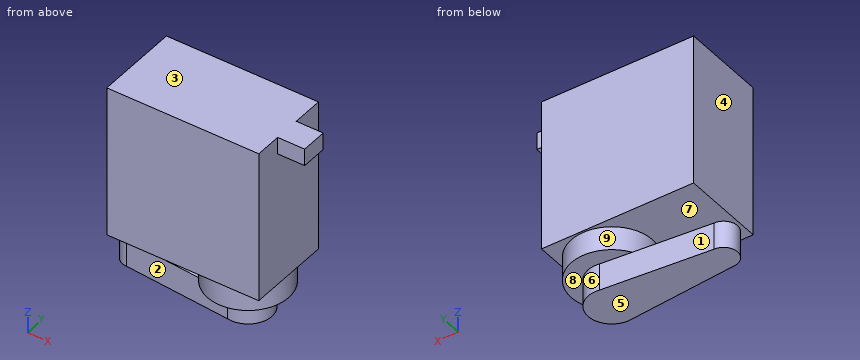
```python
from build123d import *

# Parameters (mm, degrees)
SKETCH1_W           = 22.5
SKETCH1_H           = 12.5
BOSS_EXTRUDE1_DEPTH = 22.5
SKETCH2_R           = 6
BOSS_EXTRUDE2_DEPTH = 3.5
BOSS_EXTRUDE4_DEPTH = 4
SKETCH6_W           = 2.526093831
SKETCH6_H           = 3.888015028
BOSS_EXTRUDE5_DEPTH = 4


with BuildPart() as part:
    # Sketch1 → Boss-Extrude1 (new body)
    with BuildSketch(Plane.XY):
        Rectangle(SKETCH1_W, SKETCH1_H)
    extrude(amount=BOSS_EXTRUDE1_DEPTH)

    # Sketch2 → Boss-Extrude2 (add)
    with BuildSketch(Plane(origin=(0, 0, 0), x_dir=(-1, 0, 0), z_dir=(0, 0, -1))):
        with Locations((-5.25, 0)):
            Circle(SKETCH2_R)
    extrude(amount=BOSS_EXTRUDE2_DEPTH)

    # Sketch5 → Boss-Extrude4 (add)
    with BuildSketch(Plane(origin=(0, 0, -3.5), x_dir=(-1, 0, 0), z_dir=(0, 0, -1))):
        with BuildLine():
            Line((-4.635129487, 3.455724852), (11.29, 2.05))
            ThreePointArc((11.29, 2.05), (13.34, 0), (11.29, -2.05))
            Line((11.29, -2.05), (-4.635129487, -3.455724852))
            ThreePointArc((-4.635129487, -3.455724852), (-8.76, 0), (-4.635129487, 3.455724852))
        make_face()
    extrude(amount=BOSS_EXTRUDE4_DEPTH)

    # Sketch6 → Boss-Extrude5 (add)
    with BuildSketch(Plane(origin=(11.25, 0, 0), x_dir=(0, 0, -1), z_dir=(1, 0, 0))):
        with Locations((-21.236953085, -0.353333214)):
            Rectangle(SKETCH6_W, SKETCH6_H)
    extrude(amount=BOSS_EXTRUDE5_DEPTH)


solid = part.part
```
The model under review builds one solid part; all positions refer to its coordinate system, in mm. Face numbers are marked on the shaded views. A direction names the side the tool comes from. Round coordinates to 2 decimals unless told otherwise and drop trailing zeros. Loops run counter-clockwise (first coordinate to the right, second up) from the corner with the lowest first, then second, coordinate; pieces in that order, holes last. Notation, with made-up numbers: (89.5, 42) - (94.5, 42) arc R30 ccw to (94.5, 72) - close; hole circle Ø6 at (58.25, -33.5). An arc over 180 degrees is marked (long way). Write each question's results on one line, items separated by ' | '. Start each with the question number.
Q1. Take a section at D-D on x = 10. Give the boundary of the cut face in (y, z).
Q2. Take a section at A-A on x = -2.75. Give the boundary of the cut face in (y, z), plus the area to 3 significant figures.
Q3. Wall thickness on line 1 along Z through (x, y) = (-6.5, -0.25); line 2 along X through (y, z) = (1.75, 13); line 3 along Z through (x, y) = (-10.25, 2.25): over which ranges is each line inside the solid? List them lowest first. Write a range as [from, to].
Q4. Draft analysis for pull direction Z (two halves, no side actions). For the marked faces 6, 7, 8 and 9, state which applies: pulls with the +Z half, pulls with the -Z half, needs draft (parallel to the pull), parting line crosses it, or undercut.
Q5. Take a section at B-B on z = 2. Give the boundary of the cut face in (x, y).
Q6. Tool access review of the marked faces 1, 2, 3, 4 and 5: name each direction out of +Z, -Z, +X, -X, +Y, -Y from which nothing blocks a thin tool from reaching the whole face with its end or side.
Q7. Take a section at C-C on x = 5.25. Give the boundary of the cut face in (y, z).
Q8. Insertion check: P1, Ø4, axis at y = 1.5, z = 15.5, coming from the +X side; P2, Ø2, axis at x = 13.5, z = 22, coming from the +Y side; P3, Ø3, axis at x = 13, z = 21, coming from the -Y side. Each pin has a flat end and moves straight along its axis. Give the tip position at first contact, or say it passes through.
Data:
1) outline: (-6.25, 0) - (-3.67, 0) - (-3.67, -3.5) - (3.67, -3.5) - (3.67, 0) - (6.25, 0) - (6.25, 22.5) - (-6.25, 22.5) - close
2) outline: (-6.25, 0) - (6.25, 0) - (6.25, 22.5) - (-6.25, 22.5) - close; (-2.8, -7.5) - (2.8, -7.5) - (2.8, -3.5) - (-2.8, -3.5) - close | area: 304 mm²
3) line 1: z = [-7.5, -3.5], [0, 22.5] | line 2: x = [-11.25, 11.25] | line 3: z = [0, 22.5]
4) face 6: needs draft | face 7: undercut | face 8: pulls with the -Z half | face 9: undercut
5) outline: (-11.25, -6.25) - (11.25, -6.25) - (11.25, 6.25) - (-11.25, 6.25) - close
6) face 1: -Z, -X, +Y | face 2: -Z, -X, -Y | face 3: +Z, +X, -X, +Y, -Y | face 4: +Z, -X, +Y, -Y | face 5: -Z, +X, -X, +Y, -Y
7) outline: (-6.25, 0) - (-6, 0) - (-6, -3.5) - (-3.51, -3.5) - (-3.51, -7.5) - (3.51, -7.5) - (3.51, -3.5) - (6, -3.5) - (6, 0) - (6.25, 0) - (6.25, 22.5) - (-6.25, 22.5) - close
8) P1: stops at x = 11.25 | P2: stops at y = 1.59 | P3: stops at y = -2.3
